Verification items for the finished model (mm, model axes). Face numbers are marked on the shaded views. A direction names the side the tool comes from. Round coordinates to 2 decimals unless told otherwise and drop trailing zeros. Order: outer loops, then holes, each group sorted by start corner. A loop starts at its lowest first (then second) coordinate and runs counter-clockwise, first axis right, second up. Notation, with made-up numbers: (89.5, -9) -> (132.5, -9) arc R19 ccw to (132.5, 28) -> close; hole circle Ø3 at (66.25, -13). An arc over 180 degrees is marked (long way). Return JSON: item names as keys, results as strings. Group by question number.
1) Depth check by flat-ended pin: pin 1 (10 mm diameter, centred on y = -1.5, z = 7.5, fed in from -X); pin 2 (10 mm diameter, centred on x = -15.5, y = -2.5, fed in from +Z); pin 3 (10 mm diameter, centred on y = -11, z = 46.5, fed in from +X); pin 4 (1.5 mm diameter, centred on y = 0, z = 8.5, fed in from +X). Enter the tip coordinate at first touch or a pass-through.
2) Tool access check on the marked faces 4, 5 and 6. Record the directions out of +Z, -Z, +X, -X, +Y, -Y that give a thin tool (end or side, any length) a straight path to the whole face; none if there is none.
3) Scan lines: L1, parallel to Y at x = -24, z = 63.8; L2, parallel to Z at x = -21, y = -12.75; L3, parallel to X at y = 7.25, z = 56.5. Record each from-to range of solid material in increasing order.
4) Section check C-C on x = 11.5. Enter the section's corners in (y, z), plus the area to 3 significant figures.
5) Draft check along Z on the marked faces 1, 2 and 3. Enter one of: pulls with the +Z half, pulls with the -Z half, needs draft (parallel to the pull), parting line crosses it, or undercut.
6) Section check B-B on z = 11.5. Enter the section's corners in (x, y), plus the area to 3 significant figures.
7) Section check A-A on y = -11.75. Enter the section's corners in (x, z).
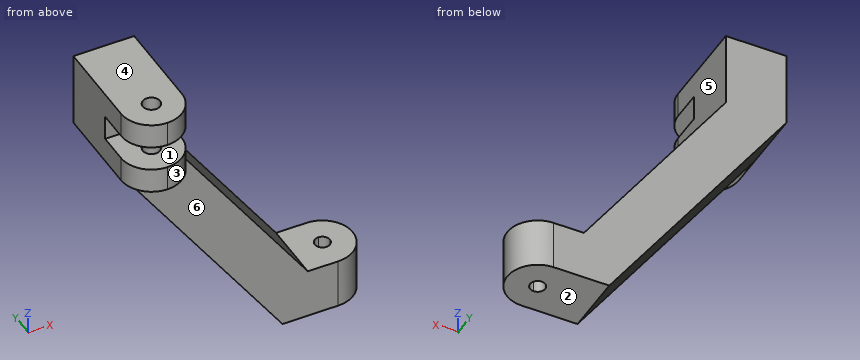
```python
from build123d import *

# Parameters (mm, degrees)
F1_DEPTH  = 20
F2_START  = 10
F1_FACE_R = 1.5
F2_DEPTH  = 10
F3_DEPTH  = 50
F5_DEPTH  = 12.001
F6_DEPTH  = 15
F7_W      = 12
F7_H      = 5
F8_DEPTH  = 12
F9_R      = 5.99999
F11_D     = 3.4


# Not quite as in the source:
# - a fillet or chamfer is up to 0.001 mm smaller than in the source, because OpenCascade refuses the exact size
# - a feature names something its author has since deleted; it is built from what else it names


with BuildPart() as f1:
    # F0 (on Top) → F1 (new body)
    with BuildSketch(Plane.XY):
        with BuildLine():
            ThreePointArc((16, -2), (22, 4), (16, 10))
            Line((16, 10), (16, 5.5))
            ThreePointArc((16, 5.5), (17.0606601718, 5.0606601718), (17.5, 4))
            ThreePointArc((17.5, 4), (17.0606601718, 2.9393398282), (16, 2.5))
            Line((16, 2.5), (16, -2))
        make_face()
        with BuildLine():
            Line((16, 5.5), (16, 10))
            ThreePointArc((16, 10), (11.7573593129, 8.2426406871), (10, 4))
            ThreePointArc((10, 4), (11.7573593129, -0.2426406871), (16, -2))
            Line((16, -2), (16, 2.5))
            ThreePointArc((16, 2.5), (14.5, 4), (16, 5.5))
        make_face()
        with BuildLine():
            Line((16, 10), (10, 10))
            Line((10, 10), (10, 4))
            ThreePointArc((10, 4), (11.7573593129, 8.2426406871), (16, 10))
        make_face()
        with BuildLine():
            ThreePointArc((16, -2), (11.7573593129, -0.2426406871), (10, 4))
            Line((10, 4), (10, -2))
            Line((10, -2), (16, -2))
        make_face()
    extrude(amount=F1_DEPTH)

    # F0 (on Top) + F1_face (on face) → F2 (cut)
    with BuildSketch(Plane.XY.offset(F2_START)):
        with BuildLine():
            ThreePointArc((16, -2), (22, 4), (16, 10))
            Line((16, 10), (16, 5.5))
            ThreePointArc((16, 5.5), (17.0606601718, 5.0606601718), (17.5, 4))
            ThreePointArc((17.5, 4), (17.0606601718, 2.9393398282), (16, 2.5))
            Line((16, 2.5), (16, -2))
        make_face()
        with BuildLine():
            Line((16, 5.5), (16, 10))
            ThreePointArc((16, 10), (11.7573593129, 8.2426406871), (10, 4))
            ThreePointArc((10, 4), (11.7573593129, -0.2426406871), (16, -2))
            Line((16, -2), (16, 2.5))
            ThreePointArc((16, 2.5), (14.5, 4), (16, 5.5))
        make_face()
        with BuildLine():
            ThreePointArc((16, -2), (11.7573593129, -0.2426406871), (10, 4))
            Line((10, 4), (10, -2))
            Line((10, -2), (16, -2))
        make_face()
        with BuildLine():
            Line((16, 10), (10, 10))
            Line((10, 10), (10, 4))
            ThreePointArc((10, 4), (11.7573593129, 8.2426406871), (16, 10))
        make_face()
    with BuildSketch(Plane(origin=(15.4073102565, 4, 20), x_dir=(1, 0, 0), z_dir=(0, 0, 1)).offset(F2_START)):
        with BuildLine():
            ThreePointArc((0.5926897435, -6), (6.5926897435, 0), (0.5926897435, 6))
            Line((0.5926897435, 6), (-5.4073102565, 6))
            Line((-5.4073102565, 6), (-5.4073102565, -6))
            Line((-5.4073102565, -6), (0.5926897435, -6))
        make_face()
        with Locations((0.5926897435, 0)):
            Circle(F1_FACE_R, mode=Mode.SUBTRACT)
    extrude(amount=F2_DEPTH, mode=Mode.SUBTRACT)

    # F0 (on Top) → F3 (join)
    with BuildSketch(Plane.XY):
        Polygon((10, 4), (10, 10), (-30, 10), (-30, -2), (10, -2), align=None)
    extrude(amount=F3_DEPTH)

    # F4 (on face) → F5 (cut, through all)
    with BuildSketch(Plane(origin=(0, 10, 0), x_dir=(-1, 0, 0), z_dir=(0, 1, 0))):
        Polygon((-10, 50), (-10, 10), (18, 50), align=None)
        Polygon((30, 0), (30, 50), (-5, 0), align=None)
    extrude(amount=-F5_DEPTH, mode=Mode.SUBTRACT)

    # F6 (add): a face of the model
    f6_faces = [f1.faces().sort_by_distance(p)[0] for p in [
        (-24, 4, 50),
    ]]
    extrude(f6_faces, amount=F6_DEPTH)

    # F7 (on face) → F8 (join)
    with BuildSketch(Plane.XZ.offset(2)):
        with Locations((-24, 52.5)):
            Rectangle(F7_W, F7_H)
        with Locations((-24, 62.5)):
            Rectangle(F7_W, F7_H)
    extrude(amount=F8_DEPTH)

    # F9 (radius 6 in the source; OpenCascade refuses exactly that, so slightly less here)
    f9_edges = [f1.edges().sort_by_distance(p)[0] for p in [
        (-30, -14, 62.5),
        (-18, -14, 62.5),
        (-18, -14, 52.5),
        (-30, -14, 52.5),
    ]]
    fillet(f9_edges, radius=F9_R)

    # F11 (through all)
    with Locations(Plane.XY.offset(65)):
        with Locations((-24, -8)):
            Hole(F11_D / 2)


solid = f1.part
```
Check result:
{
 "1": {"pin 1": "x = -3.75", "pin 2": "z = 65", "pin 3": "x = -18", "pin 4": "x = 21.04"},
 "2": {"face 4": "+Z, +X, -X, +Y, -Y", "face 5": "+Z, +X, +Y, -Y", "face 6": "-Z, +X, -X, -Y"},
 "3": {"L1": "-14 to -9.7, -6.3 to 10", "L2": "50 to 55, 60 to 65", "L3": "-30 to -18"},
 "4": {"outline": "(-2, 0) -> (10, 0) -> (10, 10) -> (-2, 10) -> close", "area": "120 mm^2"},
 "5": {"face 1": "undercut", "face 2": "pulls with the -Z half", "face 3": "needs draft"},
 "6": {"outline": "(-3.05, -2) -> (8.95, -2) -> (8.95, 10) -> (-3.05, 10) -> close", "area": "144 mm^2"},
 "7": {"outline": "(-28.68, 50) -> (-19.32, 50) -> (-19.32, 55) -> (-28.68, 55) -> close; (-28.68, 60) -> (-19.32, 60) -> (-19.32, 65) -> (-28.68, 65) -> close"}
}
